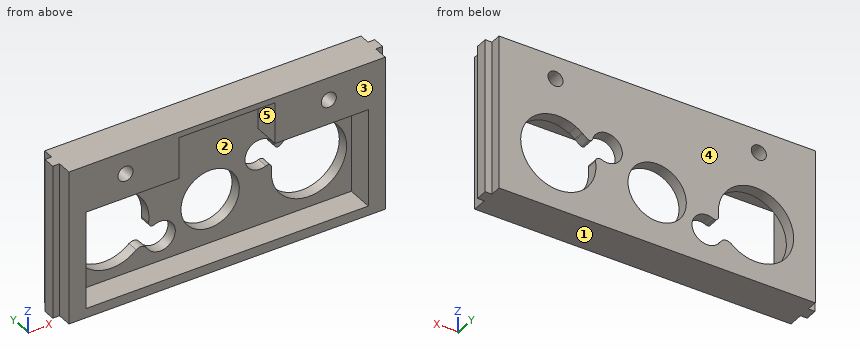
from build123d import *

# Parameters (mm, degrees)
SKETCH1_W                   = 75
SKETCH1_H                   = 26.5
BASE_01_DEPTH               = 10
SKETCH4_R                   = 7.75
SKETCH4_R_2                 = 10
SKETCH4_R_3                 = 4
CAMERA_LIGHTS_DEPTH         = 42.00990734
SKETCH5_W                   = 75
SKETCH5_H                   = 10
UPPER_SIDE_SUPPORT_DEPTH    = 5
SKETCH6_W                   = 31.5
SKETCH6_H                   = 10
LEFT_SIDE_SUPPORT_DEPTH     = 4.5
SKETCH7_W                   = 31.5
SKETCH7_H                   = 10
RIGHT_SIDE_SUPPORT_DEPTH    = 4.5
SKETCH8_W                   = 75
SKETCH8_H                   = 2.5
BASE_01_CUT_DEPTH           = 7
SKETCH10_W                  = 31.5
SKETCH10_H                  = 3.2
LEFT_SIDE_BODY_HOLDER_DEPTH = 1.8
LOWER_BASE_SUPPORT_DEPTH    = 9.5
SKETCH12_W                  = 25.5
SKETCH12_H                  = 7
CAMERA_WIRE_EXT_CUT_DEPTH   = 1.5
SKETCH13_R                  = 2
CAMERA_HOLDING_HOLES_DEPTH  = 51.35873807
IR_START                    = -3
IR_FIT_CUT_DEPTH            = 3
IR_FIT_CUT_2_DEPTH          = 3


# Read off the part's stored shape, not the designer's step: IR Fit Cut
with BuildPart() as part:
    # Sketch1 → Base 01 (new body)
    with BuildSketch(Plane(origin=(0, 0, 0), x_dir=(1, 0, 0), z_dir=(0, 1, 0))):
        Rectangle(SKETCH1_W, SKETCH1_H)
    extrude(amount=BASE_01_DEPTH)

    # Sketch4 → Camera & lights (cut, through all)
    with BuildSketch(Plane(origin=(0, 10, 0), x_dir=(1, 0, 0), z_dir=(0, 1, 0))):
        with Locations(Location((0, 4, 0), (0, 0, 270))):
            Circle(SKETCH4_R)
        with Locations(Location((-26.25, 3, 0), (0, 0, 270))):
            Circle(SKETCH4_R_2)
        with Locations(Location((26.25, 3, 0), (0, 0, 90))):
            Circle(SKETCH4_R_2)
        with Locations(Location((-13.25, 9.15, 0), (0, 0, 270))):
            Circle(SKETCH4_R_3)
        with Locations(Location((13.25, -3.15, 0), (0, 0, 270))):
            Circle(SKETCH4_R_3)
    extrude(amount=-CAMERA_LIGHTS_DEPTH, mode=Mode.SUBTRACT)

    # Sketch5 → Upper side support (add)
    with BuildSketch(Plane(origin=(0, 0, -13.25), x_dir=(-1, 0, 0), z_dir=(0, 0, -1))):
        with Locations((0, 5)):
            Rectangle(SKETCH5_W, SKETCH5_H)
    extrude(amount=UPPER_SIDE_SUPPORT_DEPTH)

    # Sketch6 → Left Side Support (add)
    with BuildSketch(Plane.ZY.offset(37.5)):
        with Locations((-2.5, 5)):
            Rectangle(SKETCH6_W, SKETCH6_H)
    extrude(amount=LEFT_SIDE_SUPPORT_DEPTH)

    # Sketch7 → Right Side Support (add)
    with BuildSketch(Plane(origin=(37.5, 0, 0), x_dir=(0, 0, -1), z_dir=(1, 0, 0))):
        with Locations((2.5, 5)):
            Rectangle(SKETCH7_W, SKETCH7_H)
    extrude(amount=RIGHT_SIDE_SUPPORT_DEPTH)

    # Sketch8 → Base 01 Cut (cut)
    with BuildSketch(Plane.XZ):
        with Locations((0, -14.5)):
            Rectangle(SKETCH8_W, SKETCH8_H)
        Polygon((-37.5, 10.25), (-37.5, -13.25), (37.5, -13.25), (37.5, 10.25), (12.75, 10.25), (12.75, 13.25), (-12.75, 13.25), (-12.75, 10.25), align=None)
    extrude(amount=-BASE_01_CUT_DEPTH, mode=Mode.SUBTRACT)

    # Sketch10 → Left Side body Holder (add)
    with BuildSketch(Plane.ZY.offset(42)):
        with Locations((-2.5, 5.5)):
            Rectangle(SKETCH10_W, SKETCH10_H)
    left_side_body_holder = extrude(amount=LEFT_SIDE_BODY_HOLDER_DEPTH)

    # Right Side body Holder: Left Side body Holder across plane
    add(left_side_body_holder.mirror(Plane(origin=(0, 0, 0), x_dir=(0, 0, 1), z_dir=(1, 0, 0))))

    # Sketch11 → Lower base support (add)
    with BuildSketch(Plane.XY.offset(13.25)):
        Polygon((42, 3.9), (43.8, 3.9), (43.8, 7.1), (42, 7.1), (42, 10), (-42, 10), (-42, 7.1), (-43.8, 7.1), (-43.8, 3.9), (-42, 3.9), (-42, 0), (-12.75, 0), (-12.75, 7), (12.75, 7), (12.75, 0), (42, 0), align=None)
    extrude(amount=LOWER_BASE_SUPPORT_DEPTH)

    # Sketch12 → Camera Wire Ext cut (add)
    with BuildSketch(Plane.XY.offset(22.75)):
        with Locations((0, 3.5)):
            Rectangle(SKETCH12_W, SKETCH12_H)
    extrude(amount=-CAMERA_WIRE_EXT_CUT_DEPTH)

    # Sketch13 → Camera Holding Holes (cut, through all)
    with BuildSketch(Plane.XZ):
        with Locations(Location((27, 16.75, 0), (0, 0, 270))):
            Circle(SKETCH13_R)
        with Locations(Location((-27, 16.75, 0), (0, 0, 270))):
            Circle(SKETCH13_R)
    extrude(amount=-CAMERA_HOLDING_HOLES_DEPTH, mode=Mode.SUBTRACT)

    # IR Fit Cut outline → IR Fit Cut (cut)
    with BuildSketch(Plane(origin=(0, 10, 0), x_dir=(1, 0, 0), z_dir=(0, 1, 0)).offset(IR_START)):
        with BuildLine():
            ThreePointArc((14.81661521, 0.530450623), (16.802776188, -1.31212586), (17.159118071, -3.99781832))
            add(Edge.make_bspline(
                [(17.159118071, -3.99781832), (17.166278119, -3.969934013), (17.178337476, -3.936891555), (17.246780801, -3.833932894), (17.305076574, -3.770665125), (17.4349321, -3.591329111), (17.910202533, -3.389398307), (18.485343295, -3.51410072), (19.253649785, -4.184734467), (19.696093453, -4.554177367), (19.740193994, -4.590943668)],
                knots=[0.275674193, 0.275674193, 0.275674193, 0.275674193, 0.290109149, 0.298316137, 0.344073007, 0.355594369, 0.407810154, 0.509906244, 0.719358573, 0.742631054, 0.742631054, 0.742631054, 0.742631054], degree=3))
            ThreePointArc((19.740193994, -4.590943668), (17.497995952, -1.83760531), (16.359278951, 1.525674007))
            add(Edge.make_bspline(
                [(14.81661521, 0.530450623), (15.181815782, 0.40272852), (15.86245956, 0.462037657), (16.265810628, 1.050757555), (16.365277346, 1.362969111), (16.359278951, 1.525674007)],
                knots=[0.222395894, 0.222395894, 0.222395894, 0.222395894, 0.382891887, 0.477494733, 0.530327084, 0.530327084, 0.530327084, 0.530327084], degree=3))
        make_face()
        with BuildLine():
            ThreePointArc((21.469612645, -5.783387543), (20.701388337, -5.319429584), (19.977853966, -4.788464812))
            add(Edge.make_bspline(
                [(19.977853966, -4.788464812), (20.110594541, -4.897809063), (20.298403446, -5.048291915), (20.760469103, -5.372959062), (21.111213366, -5.596213213), (21.469612645, -5.783387543)],
                knots=[0.784128545, 0.784128545, 0.784128545, 0.784128545, 0.852708708, 0.878445602, 1, 1, 1, 1], degree=3))
        make_face()
        with BuildLine():
            ThreePointArc((-19.618250253, 10.484643966), (-17.433842543, 7.71967877), (-16.344107974, 4.368686656))
            add(Edge.make_bspline(
                [(-16.344107974, 4.368686656), (-16.346786074, 4.400652489), (-16.363410494, 4.682682191), (-16.259037035, 4.912025365), (-16.023124853, 5.263934466), (-15.852731431, 5.462556558), (-15.60349989, 5.608912133), (-15.554028579, 5.614463051), (-15.094185027, 5.582253589), (-15.041983124, 5.573857318)],
                knots=[0.560427253, 0.560427253, 0.560427253, 0.560427253, 0.567434759, 0.623494809, 0.639172793, 0.708536611, 0.730178495, 0.833949751, 0.846921158, 0.846921158, 0.846921158, 0.846921158], degree=3))
            ThreePointArc((-15.041983124, 5.573857318), (-17.118345184, 8.132205554), (-16.569932259, 11.381154364))
            add(Edge.make_bspline(
                [(-19.618250253, 10.484643966), (-19.339728391, 10.325698426), (-18.991295195, 10.23044062), (-18.442190237, 10.020965988), (-17.459671267, 10.214555154), (-16.971941729, 10.950254946), (-17.098342068, 10.607973515), (-16.595700977, 11.343869746), (-16.569932259, 11.381154364)],
                knots=[0.533161585, 0.533161585, 0.533161585, 0.533161585, 0.632900245, 0.655820771, 0.750528398, 0.776212567, 0.886978295, 0.892604255, 0.892604255, 0.892604255, 0.892604255], degree=3))
        make_face()
    extrude(amount=IR_FIT_CUT_DEPTH, mode=Mode.SUBTRACT)

    # IR Fit Cut 2 outline → IR Fit Cut 2 (add)
    with BuildSketch(Plane(origin=(0, 10, 0), x_dir=(1, 0, 0), z_dir=(0, 1, 0)).offset(IR_START)):
        with BuildLine():
            add(Edge.make_bspline(
                [(19.740193994, -4.590943668), (19.76337103, -4.610266194), (19.841872549, -4.675657908), (19.921206817, -4.741802064), (19.977853966, -4.788464812)],
                knots=[0.742631054, 0.742631054, 0.742631054, 0.742631054, 0.754861905, 0.784128545, 0.784128545, 0.784128545, 0.784128545], degree=3))
            ThreePointArc((19.740193994, -4.590943668), (19.858260946, -4.690622333), (19.977853966, -4.788464812))
        make_face()
    extrude(amount=IR_FIT_CUT_2_DEPTH)


solid = part.part
Model file for the job. Use its own axes, mm. Face numbers are marked on the shaded views. A direction names the side the tool comes from. Give positions to 0.01 mm unless a question says otherwise; leave off trailing zeros. Order: outer loops, then holes, each group sorted by start corner. A loop starts at its lowest first (then second) coordinate and runs counter-clockwise, first axis right, second up. Notation, with made-up numbers: (40.5, 88.25) -> (59.5, 88.25) arc R17 ccw to (59.5, 107.25) -> close; hole circle Ø1 at (-5, 12.25). An arc over 180 degrees is marked (long way). Use CSV: the item, a comma, the result in double quotes.
1. Drop flat-ended pins along their axis: pin 1 (4.5 mm diameter, centred on y = 1.5, z = -3, fed in from +X); pin 2 (0.5 mm diameter, centred on x = 43.5, z = 11, fed in from +Y); pin 3 (10 mm diameter, centred on x = -5.5, z = 10, fed in from -Y). Give the stop position or say it passes through.
Outcome:
pin 1,"x = 42"
pin 2,"y = 7.1"
pin 3,"y = 7"
2. Band-saw the part on B-B, the plane z = -3. Give the cut face in (x, y).
Outcome:
outline,"(-43.8, 3.9) -> (-42, 3.9) -> (-42, 0) -> (-37.5, 0) -> (-37.5, 7) -> (-36.25, 7) -> (-36.25, 10) -> (-42, 10) -> (-42, 7.1) -> (-43.8, 7.1) -> close; (-16.25, 7) -> (-7.69, 7) -> (-7.69, 10) -> (-16.25, 10) -> close; (7.69, 7) -> (16.25, 7) -> (16.25, 10) -> (7.69, 10) -> close; (36.25, 7) -> (37.5, 7) -> (37.5, 0) -> (42, 0) -> (42, 3.9) -> (43.8, 3.9) -> (43.8, 7.1) -> (42, 7.1) -> (42, 10) -> (36.25, 10) -> close"
3. Band-saw the part on D-D, the plane z = 16.5. Give the cut face in (x, y), then the cut area to 3 significant figures.
Outcome:
outline,"(-43.8, 3.9) -> (-42, 3.9) -> (-42, 0) -> (-28.98, 0) -> (-28.98, 10) -> (-42, 10) -> (-42, 7.1) -> (-43.8, 7.1) -> close; (-25.02, 0) -> (-12.75, 0) -> (-12.75, 7) -> (12.75, 7) -> (12.75, 0) -> (25.02, 0) -> (25.02, 10) -> (-25.02, 10) -> close; (28.98, 0) -> (42, 0) -> (42, 3.9) -> (43.8, 3.9) -> (43.8, 7.1) -> (42, 7.1) -> (42, 10) -> (28.98, 10) -> close"
area,"594 mm²"
4. Mould opens along Z. For the marked faces 1, 2 and 3 say: +Z half, -Z half, draft (parallel to the pull), parting line (faces both ways), or undercut.
Outcome:
face 1,"-Z half"
face 2,"undercut"
face 3,"draft"
5. Drill centre lines: line 1 along X through (y, z) = (4.25, 16.75); line 2 along X through (y, z) = (2.5, 16.75); line 3 along Z through (x, y) = (13, 5.5). Where is each one in solid material? Low to high. Write a range as from..to.
Outcome:
line 1,"-43.8..-29, -25..-12.75, 12.75..25, 29..43.8"
line 2,"-42..-29, -25..-12.75, 12.75..25, 29..42"
line 3,"-18.25..-15.75, 10.25..22.75"
6. Band-saw the part on C-C, the plane x = 27. Give the cut face in (y, z).
Outcome:
outline,"(0, -18.25) -> (10, -18.25) -> (10, -12.97) -> (7, -12.97) -> (7, -15.75) -> (0, -15.75) -> close; (0, 10.25) -> (7, 10.25) -> (7, 6.97) -> (10, 6.97) -> (10, 14.75) -> (0, 14.75) -> close; (0, 18.75) -> (10, 18.75) -> (10, 22.75) -> (0, 22.75) -> close"
7. Band-saw the part on A-A, the plane y = 6. Give the cut face in (x, z).
Outcome:
outline,"(-43.8, -18.25) -> (43.8, -18.25) -> (43.8, 22.75) -> (-43.8, 22.75) -> close; hole (-37.5, -15.75) -> (37.5, -15.75) -> (37.5, 10.25) -> (12.75, 10.25) -> (12.75, 21.25) -> (-12.75, 21.25) -> (-12.75, 10.25) -> (-37.5, 10.25) -> close; hole circle Ø4 at (-27, 16.75); hole circle Ø4 at (27, 16.75)"
8. 3-axis set-ups, long thin cutter, end or side, ignore diameter. For the marked faces 4 and 5: which of +Z, -Z, +X, -X, +Y, -Y reach the whole face in a straight line?
Outcome:
face 4,"+Z, -Z, +X, -X, +Y"
face 5,"-Y"
